```python
from build123d import *

# Parameters (mm, degrees)
F1_DEPTH = 63.5
F0_W     = 25.4
F0_H     = 19.05
F0_H_2   = 4.7498
F0_H_3   = 4.7752
F2_DEPTH = 25.4
F4_DEPTH = 3.175
F5_R     = 12.7


with BuildPart() as f1:
    # F0 (on Front) → F1 (new body, symmetric)
    with BuildSketch(Plane.XZ):
        Polygon((-41.275, -9.525), (41.275, -9.525), (41.275, 9.525), (22.225, 9.525), (-41.275, 9.525), align=None)
    extrude(amount=F1_DEPTH, both=True)

    # F0 (on Front) → F2 (join, symmetric)
    with BuildSketch(Plane.XZ):
        with BuildLine():
            Line((22.225, 9.525), (41.275, 9.525))
            Line((41.275, 9.525), (41.275, 27.0002))
            ThreePointArc((41.275, 27.0002), (45.9246798487, 38.2255201513), (57.15, 42.8752))
            Line((57.15, 42.8752), (60.325, 42.8752))
            Line((60.325, 42.8752), (60.325, 61.9252))
            Line((60.325, 61.9252), (57.15, 61.9252))
            add(Edge.make_bspline(
                [(54.6251217416, 61.8338132892), (55.4640803854, 61.8685780106), (56.3057470428, 61.8990488271), (57.15, 61.9252)],
                knots=[109.7820212307, 109.7820212307, 109.7820212307, 109.7820212307, 111.5045361635, 111.5045361635, 111.5045361635, 111.5045361635], degree=3))
            ThreePointArc((54.6251217416, 61.8338132892), (31.5771921939, 50.7864802033), (22.225, 27.0002))
            Line((22.225, 27.0002), (22.225, 9.525))
        make_face()
        with Locations((73.025, 52.4002)):
            Rectangle(F0_W, F0_H)
        with Locations((73.025, 64.3001)):
            Rectangle(F0_W, F0_H_2)
        with Locations((73.025, 40.4876)):
            Rectangle(F0_W, F0_H_3)
    extrude(amount=F2_DEPTH, both=True)

    # F0 (on Front) → F3 (revolve)
    with BuildSketch(Plane.XZ):
        Polygon((85.725, 61.9252), (85.725, 42.8752), (85.725, 38.1), (111.125, 38.1), (111.125, 66.675), (85.725, 66.675), align=None)
    revolve(axis=Axis((85.725, 0, 52.3875), (0, 0, 1)))

    # F0 (on Front) → F4 (join, symmetric)
    with BuildSketch(Plane.XZ):
        with BuildLine():
            add(Edge.make_bspline(
                [(-41.275, 9.525), (-41.3146686629, 39.9607514864), (1.1552946366, 59.618133583), (54.6251217416, 61.8338132892)],
                knots=[0, 0, 0, 0, 109.7820212307, 109.7820212307, 109.7820212307, 109.7820212307], degree=3))
            Line((-41.275, 9.525), (22.225, 9.525))
            Line((22.225, 9.525), (22.225, 27.0002))
            ThreePointArc((22.225, 27.0002), (31.5771921939, 50.7864802033), (54.6251217416, 61.8338132892))
        make_face()
    extrude(amount=F4_DEPTH, both=True)

    # F5
    f5_edges = [f1.edges().sort_by_distance(p)[0] for p in [
        (85.725, 25.4, 52.3875),
        (73.025, 25.4, 66.675),
        (73.025, -25.4, 66.675),
        (111.125, 0, 66.675),
    ]]
    fillet(f5_edges, radius=F5_R)


solid = f1.part
```
Source: CAD feature listing. Evaluate the final solid. Frame: model axes, mm. A direction names the side the tool comes from. Give positions to 0.01 mm unless a question says otherwise; leave off trailing zeros. Loops run counter-clockwise (first coordinate to the right, second up) from the corner with the lowest first, then second, coordinate; pieces in that order, holes last. Notation, with made-up numbers: (-29.75, 24.25) -> (-16.75, 24.25) arc R27 ccw to (-16.75, 52.25) -> close; hole circle Ø2 at (5.25, 54.25). An arc over 180 degrees is marked (long way). Use a Markdown table: item, result. Add a question column.
(1) Access query for faces 1 (the face through (46, 25.4, 42)), 2 (the face through (45.8, -0.4, 38.1)), 3 (the face through (86, 0, 38.1)), 4 (the face through (22.225, 14, 18)). Directions: +Z, -Z, +X, -X, +Y, -Y. A direction counts if a zero-diameter tool reaches every point of the face in a straight line with its end or side. Return the directions, or none.
(2) Section query A-A (z = -4). Output: boundary loops of the cut face in (x, y) (3 decimals), then the cut area to 3 significant figures.
(3) Ray query, line 1 (X direction, y = 22.5, z = 24) (3 decimals); line 2 (X direction, y = -40, z = 0) (3 decimals); line 3 (Y direction, x = 20, z = 48) (3 decimals). Return the intervals inside material, ascending.
(4) First-contact query: pin 1 Ø5 at (y, z) = (-17.5, 16.5) entering from -X (3 decimals); pin 2 Ø15.5 at (x, z) = (27.5, 37) entering from -Y; pin 3 Ø2.5 at (x, y) = (58.5, -11) entering from +Z. Flat tips, straight axial feed; report the tip coordinate or a pass-through.
Checked values:
| question | item | result |
|---|---|---|
| 1 | face 1 | +Z, +X, -X, +Y |
| 1 | face 2 | -Z, +Y, -Y |
| 1 | face 3 | -Z, +X, +Y, -Y |
| 1 | face 4 | +Z, -X, +Y |
| 2 | outline | (-41.275, -63.5) -> (41.275, -63.5) -> (41.275, 63.5) -> (-41.275, 63.5) -> close |
| 2 | area | 10,500 mm^2 |
| 3 | line 1 | 22.225 to 41.275 |
| 3 | line 2 | -41.275 to 41.275 |
| 3 | line 3 | -3.175 to 3.175 |
| 4 | pin 1 | x = 22.225 |
| 4 | pin 2 | y = -25.4 |
| 4 | pin 3 | z = 61.93 |
